Part print with two shaded views. Sizes in mm from the minimum x, y, z corner. A direction names the side the tool comes from. Coordinates: 2 decimals unless noted, no trailing zeros. Write each loop counter-clockwise with the first axis right and the second up, starting at its lowest first coordinate (ties: lowest second). Pieces come first, ordered by that corner, then holes. Notation, with made-up numbers: M -15,-9 L 42,-9 A23 ccw 42,28 Z; hole C 6.5,17.5 d4. An arc over 180 degrees is marked long. One line per question, with ' | ' between items. Start each with the question number.
(1) Cut at C-C (z = 208). Write the cut outline in (x, y).
(2) Tool access for the marked faces 1 and 2: list every direction of +Z, -Z, +X, -X, +Y, -Y with a clear straight run to the whole face (end or side of a thin tool).
(3) Flat gauge pins, fed straight in: pin 1 Ø10 at (y, z) = (53.5, 113) entering from +X; pin 2 Ø2 at (y, z) = (57.5, 355.5) entering from -X; pin 3 Ø6 at (x, y) = (31.5, 59) entering from +Z; pin 4 Ø1.5 at (y, z) = (35, 107) entering from -X. Where does each tip first touch, or does it go through?
(4) Wall check: probe 1 along Y at (x, z) = (41, 349.5); probe 2 along Y at (x, z) = (41, 51); probe 3 along Z at (x, y) = (30, 73). Give the ranges that are in metal, low to high.
(5) Cut at A-A (x = 41). Write the cut outline in (y, z), plus the area to 4 significant figures.
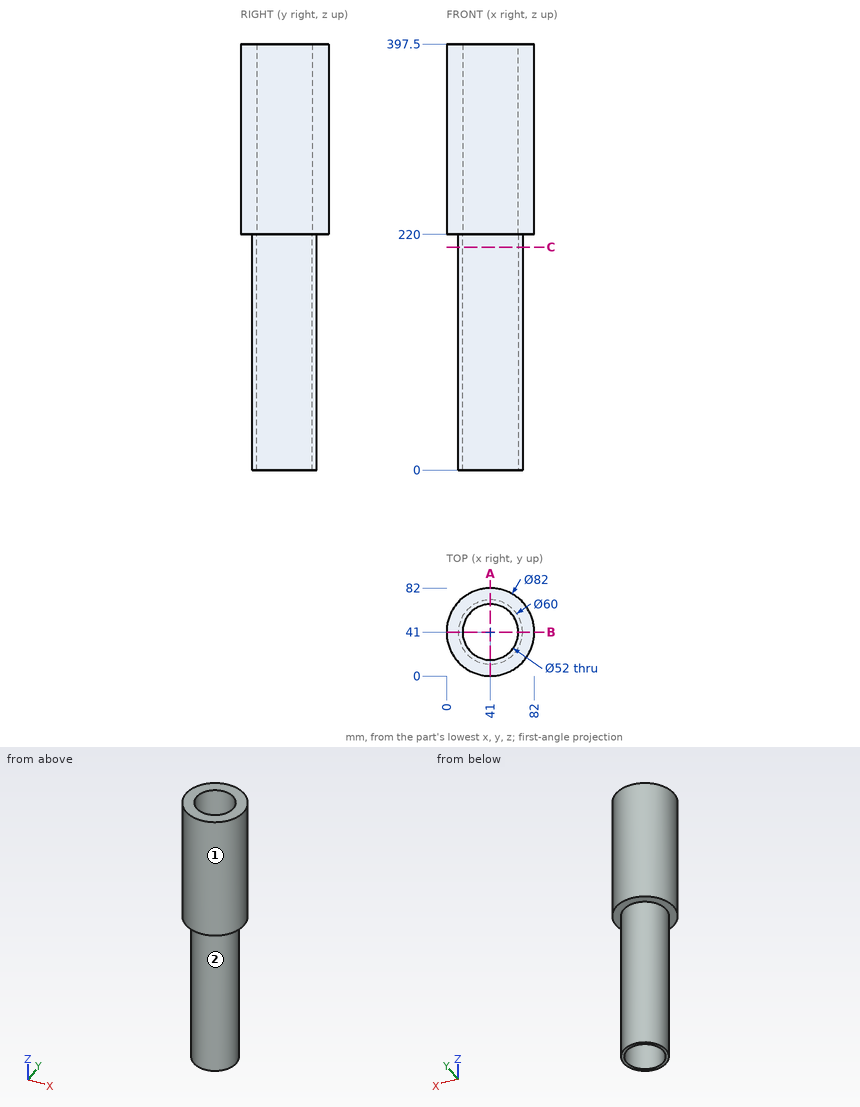
Filled in:
1) outline: C 41,41 d60; hole C 41,41 d52
2) face 1: +Z, -Z | face 2: -Z
3) pin 1: x = 70.05 | pin 2: x = 3.04 | pin 3: through | pin 4: x = 11.46
4) probe 1: 0 to 15, 67 to 82 | probe 2: 11 to 15, 67 to 71 | probe 3: 220 to 397.5
5) outline: M 0,220 L 11,220 L 11,0 L 15,0 L 15,397.5 L 0,397.5 Z; M 67,0 L 71,0 L 71,220 L 82,220 L 82,397.5 L 67,397.5 Z | area: 7,085 mm²
